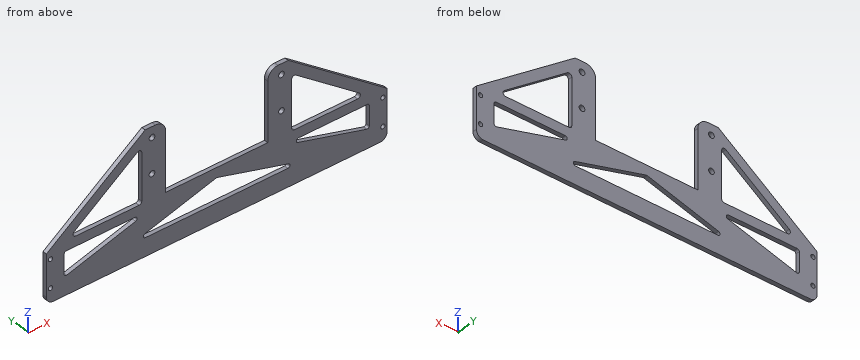
from build123d import *

# Parameters (mm, degrees)
SKETCH_1_R          = 1.6
SKETCH_1_R_2        = 2.1
EXTRUDE_1_DEPTH     = 3
FILLET_1_R          = 5
FILLET_2_R          = 7.5
CUT_EXTRUDE_1_DEPTH = 254.622258487


with BuildPart() as part:
    # 草图1 → 凸台-拉伸1 (new body)
    with BuildSketch(Plane(origin=(0, 0, 0), x_dir=(1, 0, 0), z_dir=(0, 1, 0))):
        Polygon((-3, 30), (-3, -5), (69.5, -57.5), (84.5, -57.5), (84.5, -7.5), (159.5, -7.5), (159.5, -57.5), (174.5, -57.5), (247, -5), (247, 30), align=None)
        with Locations(Location((0, 20, 0), (0, 0, 270))):
            Circle(SKETCH_1_R, mode=Mode.SUBTRACT)
        with Locations(Location((0, 0, 0), (0, 0, 270))):
            Circle(SKETCH_1_R, mode=Mode.SUBTRACT)
        with Locations(Location((244, 20, 0), (0, 0, 270))):
            Circle(SKETCH_1_R, mode=Mode.SUBTRACT)
        with Locations(Location((244, 0, 0), (0, 0, 270))):
            Circle(SKETCH_1_R, mode=Mode.SUBTRACT)
        with Locations(Location((74.5, -25, 0), (0, 0, 270))):
            Circle(SKETCH_1_R_2, mode=Mode.SUBTRACT)
        with Locations(Location((169.5, -25, 0), (0, 0, 270))):
            Circle(SKETCH_1_R_2, mode=Mode.SUBTRACT)
        with Locations(Location((74.5, -50, 0), (0, 0, 270))):
            Circle(SKETCH_1_R_2, mode=Mode.SUBTRACT)
        with Locations(Location((169.5, -50, 0), (0, 0, 270))):
            Circle(SKETCH_1_R_2, mode=Mode.SUBTRACT)
        with BuildLine():
            Line((18.559297534, -7.5), (65, -7.5))
            ThreePointArc((65, -7.5), (66.414213562, -8.085786438), (67, -9.5))
            Line((67, -9.5), (67, -43.129474199))
            ThreePointArc((67, -43.129474199), (65.909384614, -44.910771374), (63.826980376, -44.749358442))
            Line((63.826980376, -44.749358442), (17.38627791, -11.119884243))
            ThreePointArc((17.38627791, -11.119884243), (16.656698196, -8.883464716), (18.559297534, -7.5))
        make_face(mode=Mode.SUBTRACT)
        with BuildLine():
            Line((180.173019624, -44.749358442), (226.61372209, -11.119884243))
            ThreePointArc((226.61372209, -11.119884243), (227.343301804, -8.883464716), (225.440702466, -7.5))
            Line((225.440702466, -7.5), (179, -7.5))
            ThreePointArc((179, -7.5), (177.585786438, -8.085786438), (177, -9.5))
            Line((177, -9.5), (177, -43.129474199))
            ThreePointArc((177, -43.129474199), (178.090615386, -44.910771374), (180.173019624, -44.749358442))
        make_face(mode=Mode.SUBTRACT)
    extrude(amount=EXTRUDE_1_DEPTH)

    # 圆角1
    fillet_1_edges = [part.edges().sort_by_distance(p)[0] for p in [
        (247, 1.5, -30),
        (-3, 1.5, -30),
    ]]
    fillet(fillet_1_edges, radius=FILLET_1_R)

    # 圆角2
    fillet_2_edges = [part.edges().sort_by_distance(p)[0] for p in [
        (159.5, 1.5, 57.5),
        (84.5, 1.5, 57.5),
    ]]
    fillet(fillet_2_edges, radius=FILLET_2_R)

    # 草图3 → 切除-拉伸1 (cut, through all)
    with BuildSketch(Plane(origin=(0, 3, 0), x_dir=(1, 0, 0), z_dir=(0, 1, 0))):
        with BuildLine():
            Line((10, 15.02762992), (10, 1))
            ThreePointArc((10, 1), (10.439339828, -0.060660172), (11.5, -0.5))
            Line((11.5, -0.5), (62.104084647, -0.5))
            ThreePointArc((62.104084647, -0.5), (63.590394858, 0.79780713), (62.50477975, 2.445490724))
            Line((62.50477975, 2.445490724), (11.900695103, 16.473120645))
            ThreePointArc((11.900695103, 16.473120645), (10.591991921, 16.221581899), (10, 15.02762992))
        make_face()
        with BuildLine():
            Line((69.691860168, 17), (174.308139832, 17))
            ThreePointArc((174.308139832, 17), (175.794450043, 15.70219287), (174.708834935, 14.054509276))
            Line((174.708834935, 14.054509276), (122.400695103, -0.445490724))
            ThreePointArc((122.400695103, -0.445490724), (122, -0.5), (121.599304897, -0.445490724))
            Line((121.599304897, -0.445490724), (69.291165065, 14.054509276))
            ThreePointArc((69.291165065, 14.054509276), (68.205549957, 15.70219287), (69.691860168, 17))
        make_face()
        with BuildLine():
            Line((232.5, -0.5), (181.895915353, -0.5))
            ThreePointArc((181.895915353, -0.5), (180.409605142, 0.79780713), (181.49522025, 2.445490724))
            Line((181.49522025, 2.445490724), (232.099304897, 16.473120645))
            ThreePointArc((232.099304897, 16.473120645), (233.408008079, 16.221581899), (234, 15.02762992))
            Line((234, 15.02762992), (234, 1))
            ThreePointArc((234, 1), (233.560660172, -0.060660172), (232.5, -0.5))
        make_face()
    extrude(amount=-CUT_EXTRUDE_1_DEPTH, mode=Mode.SUBTRACT)


solid = part.part
Can you work these out from the model? Positions are in its coordinate system, mm. Give positions to 0.01 mm unless a question says otherwise; leave off trailing zeros. Order: outer loops, then holes, each group sorted by start corner. A loop starts at its lowest first (then second) coordinate and runs counter-clockwise, first axis right, second up. Notation, with made-up numbers: M 1,43 L 29,43 A19 ccw 29,54 Z; hole C 28,5.5 d2. An arc over 180 degrees is marked long. Use one line per item in the form item = value. Start each with the question number.
Item 1: If we section it at B-B (y = 1.25): State how many separate pieces and enclosed holes the cut face has, then the cut area to 3 significant figures.
Item 2: Will these pins go through, and if not, where does the flat tip stop? pin 1 Ø1.5 at (y, z) = (2, 21) entering from -X; pin 2 Ø0.9 at (y, z) = (1, 25.5) entering from -X; pin 3 Ø0.9 at (y, z) = (1.5, 31.5) entering from -X.
Item 3: If we section it at A-A (z = 37.5): Write out the boundary of the cut face in (x, y), then the cut area to 3 significant figures.
Item 4: If I drill on line 1 along X through (y, z) = (2.15, -20); line 2 along X through (y, z) = (2.35, 38); line 3 along Z through (x, y) = (169.5, 1.3), over which ranges is the centre line in solid material (lowest first)?
Outcome:
q1.separate_pieces = 1
q1.enclosed_holes = 13
q1.area = 9,900 mm2
q2.pin_1 = 18.06
q2.pin_2 = 24.69
q2.pin_3 = 32.97
q3.outline = M 41.88,0 L 53.82,0 L 53.82,3 L 41.88,3 Z; M 67,0 L 84.5,0 L 84.5,3 L 67,3 Z; M 159.5,0 L 177,0 L 177,3 L 159.5,3 Z; M 190.18,0 L 202.12,0 L 202.12,3 L 190.18,3 Z
q3.area = 177 mm2
q4.line_1 = -3 to -1.6, 1.6 to 242.4, 245.6 to 247
q4.line_2 = 42.57 to 54.51, 67 to 84.5, 159.5 to 177, 189.49 to 201.43
q4.line_3 = -30 to -17, -12.61 to 22.9, 27.1 to 47.9, 52.1 to 57.5
